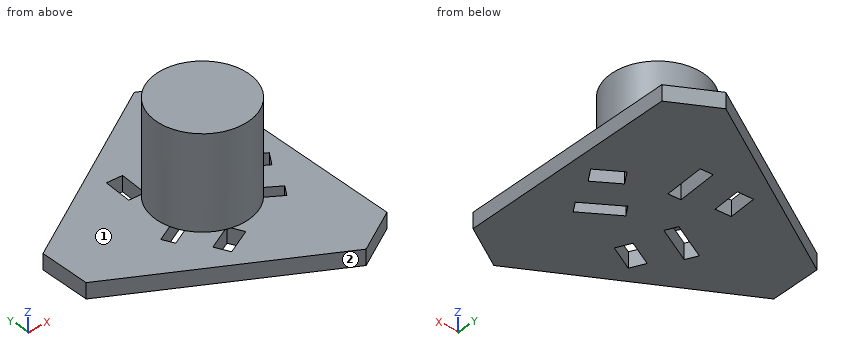
```python
from build123d import *

# Parameters (mm, degrees)
BOSS_EXTRUDE1_DEPTH = 5
CUT_EXTRUDE7_DEPTH  = 6
CIRPATTERN1_COUNT   = 3
SKETCH11_R          = 15
BOSS_EXTRUDE2_DEPTH = 30


with BuildPart() as part:
    # Sketch1 → Boss-Extrude1 (new body)
    with BuildSketch(Plane.XY):
        Polygon((-45.033320997, -8), (-45.033320997, 8), (15.588457268, 43), (29.444863729, 35), (29.444863729, -35), (15.588457268, -43), align=None)
    extrude(amount=BOSS_EXTRUDE1_DEPTH)

    # Sketch9 → Cut-Extrude7 (cut, through all)
    with BuildSketch(Plane.XY.offset(5)):
        Polygon((-19.556667785, -6.732996787), (-7.875286887, -1.028144438), (-6.119947703, -4.622415484), (-17.801328601, -10.327267832), align=None)
        Polygon((-12.054679914, -17.536708093), (-3.967570061, -13.587194928), (-1.773396081, -18.080033735), (-9.860505933, -22.029546899), align=None)
    cut_extrude7 = extrude(amount=-CUT_EXTRUDE7_DEPTH, mode=Mode.SUBTRACT)

    # CirPattern1: Cut-Extrude7 ×3 about axis
    cirpattern1_axis = Axis((0, 0, 0), (0, 0, 1))
    for i in range(1, CIRPATTERN1_COUNT):
        add(cut_extrude7.rotate(cirpattern1_axis, i * 360 / CIRPATTERN1_COUNT), mode=Mode.SUBTRACT)

    # Sketch11 → Boss-Extrude2 (add)
    with BuildSketch(Plane.XY.offset(5)):
        Circle(SKETCH11_R)
    extrude(amount=BOSS_EXTRUDE2_DEPTH)


solid = part.part
```
Geometry check sheet. Reference: the model listing, model coordinates, mm. Face numbers are marked on the shaded views. A direction names the side the tool comes from. Give positions to 0.01 mm unless a question says otherwise; leave off trailing zeros. Order: outer loops, then holes, each group sorted by start corner. A loop starts at its lowest first (then second) coordinate and runs counter-clockwise, first axis right, second up. Notation, with made-up numbers: (0, -24) - (53, -24) arc R26 ccw to (53, 11) - close; hole circle Ø7 at (70.5, 89). An arc over 180 degrees is marked (long way). Write item = value, one per line. Start each with the question number.
1) Section check A-A (z = 4). Count the separate pieces of the cut face and the enclosed holes in it, then the cut area to 3 significant figures.
2) Scan lines: L1, parallel to Z at x = 1, y = -15.5; L2, parallel to Y at x = -8, z = 4.5; L3, parallel to Y at x = 23.5, z = 2. Record each from-to range of solid material in increasing order.
3) Section check D-D (y = -28). Enter the section's corners in (x, z), then the cut area to 3 significant figures.
4) Gauge pin test, flat ends, axial feed: pin 1 Ø1 at (x, z) = (-5.5, 22) entering from -Y; pin 2 Ø10 at (x, z) = (15, 11) entering from +Y; pin 3 Ø1 at (x, y) = (-3, 28.5) entering from -Z; pin 4 Ø2 at (x, y) = (1.5, 12.5) entering from -Z. Record the tip position at first contact, or that the pin passes through.
5) Access from +Z, -Z, +X, -X, +Y, -Y to the whole of each face (thin tool, end or side, straight path). Record for the marked faces 1 and 2.
6) Section check B-B (y = 0). Enter the section's corners in (x, z).
7) Section check C-C (y = 25). Enter the section's corners in (x, z), then the cut area to 3 significant figures.
Geometry check:
q1.separate_pieces = 1
q1.enclosed_holes = 6
q1.area = 3,880 mm2
q2.L1 = 0 to 5
q2.L2 = -29.38 to -21.12, -15.56 to -5.54, -1.09 to 29.38
q2.L3 = -38.43 to 1.72, 2.82 to 38.43
q3.outline = (-10.39, 0) - (29.44, 0) - (29.44, 5) - (-10.39, 5) - close
q3.area = 199 mm2
q4.pin_1 = -14.14
q4.pin_2 = 11.18
q4.pin_3 = 0
q4.pin_4 = 5
q5.face_1 = +Z
q5.face_2 = +Z, -Z, -X, -Y
q6.outline = (-45.03, 0) - (18.73, 0) - (18.73, 5) - (15, 5) - (15, 35) - (-15, 35) - (-15, 5) - (-45.03, 5) - close; (22.34, 0) - (29.44, 0) - (29.44, 5) - (22.34, 5) - close
q7.outline = (-15.59, 0) - (29.44, 0) - (29.44, 5) - (-15.59, 5) - close
q7.area = 225 mm2
